Part model, mm, in its own coordinate system. Face numbers are marked on the shaded views. A direction names the side the tool comes from. Coordinates: 2 decimals unless noted, no trailing zeros. Loops run counter-clockwise (first coordinate to the right, second up) from the corner with the lowest first, then second, coordinate; pieces in that order, holes last. Notation, with made-up numbers: (52, 0.5) - (108, 0.5) arc R25 ccw to (108, 24.5) - close; hole circle Ø1 at (61, -19). An arc over 180 degrees is marked (long way). Answer as CSV lines item,"result".
Autodesk Inventor part; units mm, degrees
ref_plane "YZ Plane" through (0, 0, 0) normal (1, 0, 0) x (0, 1, 0)
ref_plane "XZ Plane" through (0, 0, 0) normal (0, 1, 0) x (-1, 0, 0)
ref_plane "XY Plane" through (0, 0, 0) normal (0, 0, 1) x (1, 0, 0)
sketch "Эскиз1" plane through (0, 0, 0) normal (0, 1, 0) x (-1, 0, 0)
  circle A0 centre (0, 0) radius 6
  dimension "d0" = 12
extrude "Выдавливание1" add sketch "Эскиз1" along normal blind 50
sketch "Эскиз2" plane through (0, 50, 0) normal (0, 1, 0) x (1, 0, 0)
  circle A0 centre (0, 0) radius 8
  dimension "d3" = 16
extrude "Выдавливание2" add sketch "Эскиз2" along normal blind 5
sketch "Эскиз3" plane through (0, 55, 0) normal (0, 1, 0) x (1, 0, 0)
  circle A0 centre (0, 0) radius 8
  circle A1 centre (4, 0) radius 3
  dimension "d6" = 6
  dimension "d7" = 4
extrude "Выдавливание3" add sketch "Эскиз3" along normal blind 5 contours A1
sketch "Эскиз4" plane through (0, 0, 0) normal (1, 0, 0) x (0, 1, 0)
  line L0 (0, 6.4352) -> (10.2146, 6.4352)
  line L1 (10.2146, 6.4352) -> (10.2146, -6.6395)
  line L2 (10.2146, -6.6395) -> (0, -6.6395)
  line L3 (0, -6.6395) -> (0, 6.4352)
  point P0 (0, 0)
extrude "Выдавливание4" add sketch "Эскиз4" along normal blind 14.5
sketch "Эскиз7" plane through (0, 0, 0) normal (0, -1, 0) x (1, 0, 0)
  circle A0 centre (12.2744, -0.1021) radius 2.0418
extrude "Выдавливание7" cut sketch "Эскиз7" against normal blind 14.5
sketch "Эскиз8" plane through (0, 0, -6.6395) normal (0, 0, -1) x (-1, 0, 0)
  circle A0 centre (-12.2507, 5.1073) radius 1.129
extrude "Выдавливание8" cut sketch "Эскиз8" against normal blind 14.5
properties part number "ось"
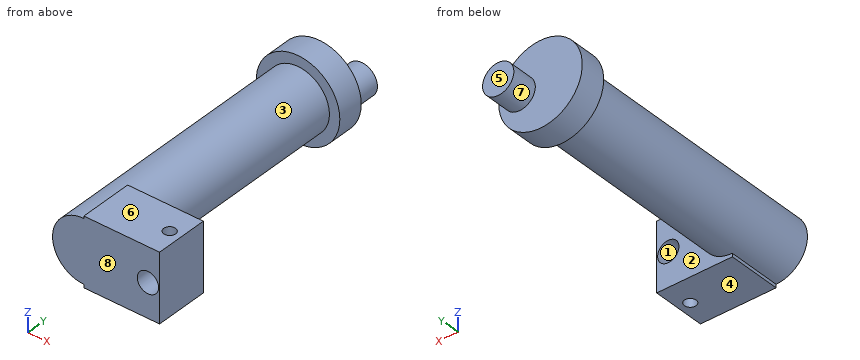
Q1. Saw through at B-B (y = 7). Give the cut face in (x, z), then the cut area to 3 significant figures.
Results:
outline,"(0, -6.64) - (14.5, -6.64) - (14.5, 6.44) - (0, 6.44) - (0, 6) arc R6 ccw to (0, -6) - close; hole circle Ø4.08 at (12.27, -0.1)"
area,"233 mm^2"
Q2. Flat gauge pins, fed straight in: pin 1 (1 mm diameter, centred on y = 25.5, z = 4.5, fed in from -X); pin 2 (8 mm diameter, centred on y = 37.5, z = -4, fed in from +X); pin 3 (5 mm diameter, centred on x = 10.5, y = 3, fed in from -Z); pin 4 (5.5 mm diameter, centred on x = 12.27, z = -0.1, fed in from -Y). Where does each tip first touch, or does it go through?
Results:
pin 1,"stops at x = -4.47"
pin 2,"stops at x = 6"
pin 3,"stops at z = -6.64"
pin 4,"stops at y = 0"
Q3. Wall check: L1, parallel to Y at x = 5.5, z = 5; L2, parallel to Z at x = 0, y = 11.5; L3, parallel to Y at x = 2, z = 7. Give the ranges that are in metal, low to high.
Results:
L1,"y = 0 to 10.21, 50 to 55"
L2,"z = -6 to 6"
L3,"y = 50 to 55"
Q4. Saw through at D-D (y = 28). Give the cut face in (x, z).
Results:
outline,"circle Ø12 at (0, 0)"
Q5. Saw through at C-C (x = 9.25). Give the cut face in (y, z), then the cut area to 3 significant figures.
Results:
outline,"(0, -6.64) - (10.21, -6.64) - (10.21, 6.44) - (0, 6.44) - close"
area,"134 mm^2"
Q6. Saw through at A-A (z = -4.5). Give the cut face in (x, y).
Results:
outline,"(-6.61, 50) - (-3.97, 50) - (-3.97, 0) - (14.5, 0) - (14.5, 10.21) - (3.97, 10.21) - (3.97, 50) - (6.61, 50) - (6.61, 55) - (-6.61, 55) - close; hole circle Ø2.26 at (12.25, 5.11)"
Q7. Which spindle directions (+Z, -Z, +X, -X, +Y, -Y) get a long thin tool onto all of the face, cutting with end or side? Do the marked faces 4, 5, 6, 7 and 8. Say none if no direction does.
Results:
face 4,"-Z, +X, -X, -Y"
face 5,"+Z, -Z, +X, -X, +Y"
face 6,"+Z, +X, -X, -Y"
face 7,"+Y"
face 8,"+Z, -Z, +X, -X, -Y"
Q8. Two-plate mould, pull along Z, no slides. Class the marked faces 1, 2 and 3: released by +Z, released by -Z, zero draft, split by the parting line, or undercut.
Results:
face 1,"undercut"
face 2,"zero draft"
face 3,"split by the parting line"
